```python
from build123d import *

# Parameters (mm, degrees)
F0_W      = 266.7
F0_H      = 98.5
F1_DEPTH  = 38
F2_R      = 47.092995
F3_DEPTH  = 1
F5_DEPTH  = 0.9
F6_W      = 0.9
F6_H      = 39.5
F7_DEPTH  = 11.3
F8_W      = 7
F8_H      = 5.4
F8_W_2    = 4.3
F8_H_2    = 3
F9_DEPTH  = 0.9
F10_W     = 94
F10_H     = 1.6
F11_DEPTH = 14


with BuildPart() as f1:
    # F0 (on Top) → F1 (new body)
    with BuildSketch(Plane.XY):
        Rectangle(F0_W, F0_H)
    extrude(amount=F1_DEPTH)

    # F2 (on face) → F3 (cut)
    with BuildSketch(Plane.XY.offset(38)):
        with Locations((-34.058255, 0.413742)):
            Circle(F2_R)
        with Locations((75.987235, 0.413742)):
            Circle(F2_R)
    extrude(amount=-F3_DEPTH, mode=Mode.SUBTRACT)

    # F4 (on face) → F5 (join)
    with BuildSketch(Plane(origin=(-133.35, 0, 0), x_dir=(0, -1, 0), z_dir=(-1, 0, 0))):
        Polygon((56.85, 38), (49.25, 38), (-49.25, 38), (-49.25, 0), (49.25, 0), (66.75, 0), (69.95, 3.2), (78.25, 3.2), (78.25, 13.5), (69.95, 13.5), (66.95, 18.5), (69.95, 23.5), (78.25, 23.5), (78.25, 33.8), (69.95, 33.8), (67.35, 36.4), (56.85, 36.4), align=None)
    extrude(amount=F5_DEPTH)

    # F6 (on face) → F7 (join)
    with BuildSketch(Plane(origin=(-134.25, 0, 0), x_dir=(0, -1, 0), z_dir=(-1, 0, 0))):
        with Locations((-43.6, 16.65)):
            Rectangle(F6_W, F6_H)
    extrude(amount=F7_DEPTH)

    # F8 (on face) → F9 (cut, through all)
    with BuildSketch(Plane(origin=(0, 44.05, 0), x_dir=(-1, 0, 0), z_dir=(0, 1, 0))):
        with Locations((137.75, -0.4)):
            Rectangle(F8_W, F8_H)
        with Locations((143.4, 26.5)):
            Rectangle(F8_W_2, F8_H_2)
        with Locations((143.4, 6.2)):
            Rectangle(F8_W_2, F8_H_2)
        with BuildLine():
            ThreePointArc((141.45, 20.4), (139.25, 22.6), (137.05, 20.4))
            Line((137.05, 20.4), (137.05, 18.9))
            ThreePointArc((137.05, 18.9), (139.25, 16.7), (141.45, 18.9))
            Line((141.45, 18.9), (141.45, 20.4))
        make_face()
    extrude(amount=-F9_DEPTH, mode=Mode.SUBTRACT)

    # F10 (on face) → F11 (join)
    with BuildSketch(Plane.XZ.offset(49.25)):
        with Locations((-40.35, 0.8)):
            Rectangle(F10_W, F10_H)
    extrude(amount=F11_DEPTH)


solid = f1.part
```
Work out the finished part from the listing and answer in its coordinate system (mm). A direction names the side the tool comes from. Round coordinates to 2 decimals unless told otherwise and drop trailing zeros. Write each loop counter-clockwise with the first axis right and the second up, starting at its lowest first coordinate (ties: lowest second). Pieces come first, ordered by that corner, then holes.
1) Consider probe 1 along Y at (x, z) = (-109.5, 6.5); probe 2 along Z at (x, y) = (-79, 16.5); probe 3 along X at (y, z) = (30.5, 30). Determine where each line is inside the solid, lowest interval first.
2) A cutting plane is placed at B-B on y = 27.5. Determine the outline of the cut face in (x, z), and give its area (3 significant figures).
3) Which of the six approach directions +Z, -Z, +X, -X, +Y, -Y give full straight-line access (tool end or side, diameter ignored) to faces 5 (the face through (-41, -56, 1.6)), 6 (the face through (-35, 1, 37)), 7 (the face through (-140, 44.05, 16))?
4) Determine the mould class of faces 1 (the face through (-140, 43.15, 16)), 2 (the face through (75, 1, 37)), 3 (the face through (133.35, -1, 19)), 4 (the face through (-68.77, 32.24, 37.51)) for opening direction Y: pulls with the +Y half, pulls with the -Y half, needs draft (parallel to the pull), parting line crosses it, or undercut.
5) A cutting plane is placed at A-A on x = 50. Determine the outline of the cut face in (y, z), and give its area (3 significant figures).
6) A cutting plane is placed at C-C on x = 105. Determine the outline of the cut face in (y, z).
7) Flat-ended cylindrical pins translate along their axes: P1, Ø0.7, axis at x = -133.5, y = -75.5, coming from the -Z side; P2, Ø9, axis at x = -142, z = 12.5, coming from the -Y side; P3, Ø11.5, axis at y = -26, z = 10, coming from the -X side. Find the tip coordinate at first contact, or state that the pin passes through.
8) A cutting plane is placed at D-D on y = -43. Determine the outline of the cut face in (x, z).
Entries:
1. probe 1: y = -49.25 to 49.25
1. probe 2: z = 0 to 38
1. probe 3: x = -134.25 to 133.35
2. outline: (-134.25, 0) - (133.35, 0) - (133.35, 38) - (114.51, 38) - (114.51, 37) - (37.46, 37) - (37.46, 38) - (4.47, 38) - (4.47, 37) - (-72.58, 37) - (-72.58, 38) - (-134.25, 38) - close
2. area: 10,000 mm2
3. face 5: +Z, +X, -Y
3. face 6: +Z
3. face 7: +Z, -Z, -X, +Y
4. face 1: pulls with the -Y half
4. face 2: undercut
4. face 3: needs draft
4. face 4: undercut
5. outline: (-49.25, 0) - (49.25, 0) - (49.25, 38) - (39.69, 38) - (39.69, 37) - (-38.86, 37) - (-38.86, 38) - (-49.25, 38) - close
5. area: 3,660 mm2
6. outline: (-49.25, 0) - (49.25, 0) - (49.25, 38) - (37.51, 38) - (37.51, 37) - (-36.68, 37) - (-36.68, 38) - (-49.25, 38) - close
7. P1: stops at z = 3.2
7. P2: stops at y = 43.15
7. P3: stops at x = -134.25
8. outline: (-134.25, 0) - (133.35, 0) - (133.35, 38) - (94.24, 38) - (94.24, 37) - (57.74, 37) - (57.74, 38) - (-15.81, 38) - (-15.81, 37) - (-52.31, 37) - (-52.31, 38) - (-134.25, 38) - close
